from build123d import *

# Parameters (mm, degrees)
F0_W     = 5
F0_H     = 50
F0_W_2   = 138.5
F0_H_2   = 20
F0_W_3   = 50
F0_H_3   = 5
F0_H_4   = 4
F0_W_4   = 20
F0_W_5   = 4
F0_H_5   = 175
F0_W_6   = 40
F0_H_6   = 40
F0_R     = 20
F1_DEPTH = 1
F0_W_7   = 128.5
F0_H_7   = 147
F2_DEPTH = 1
F3_W     = 6
F3_H     = 6
F4_DEPTH = 25


with BuildPart() as f1:
    # F0 (on Top) → F1 (new body)
    with BuildSketch(Plane.XY):
        with Locations((-231, -87.5)):
            Rectangle(F0_W, F0_H)
        with Locations((-69.25, -122.5)):
            Rectangle(F0_W_2, F0_H_2)
        with Locations((-183.5, -40)):
            Rectangle(F0_W_3, F0_H_3)
        with Locations((-69.25, 114.5)):
            Rectangle(F0_W_2, F0_H_4)
        with Locations((-218.5, -87.5)):
            Rectangle(F0_W_4, F0_H)
        with Locations((-183.5, -52.5)):
            Rectangle(F0_W_3, F0_H_2)
        with Locations((-140.5, 25)):
            Rectangle(F0_W_5, F0_H_5)
        Polygon((-138.5, -112.5), (-138.5, -62.5), (-142.5, -62.5), (-158.5, -62.5), (-158.5, -112.5), align=None)
        with Locations((-183.5, -87.5)):
            Rectangle(F0_W_3, F0_H)
        with Locations((-183.5, -87.5)):
            Rectangle(F0_W_6, F0_H_6, mode=Mode.SUBTRACT)
        Polygon((0, 102.5), (0, 112.5), (-138.5, 112.5), (-138.5, -62.5), (-138.5, -112.5), (0, -112.5), (0, -44.5), (-128.5, -44.5), (-128.5, 102.5), align=None)
        with Locations((-113.5, -87.5)):
            Circle(F0_R, mode=Mode.SUBTRACT)
    extrude(amount=F1_DEPTH)

    # F0 (on Top) → F2 (join)
    with BuildSketch(Plane.XY):
        Polygon((0, 102.5), (0, 112.5), (-138.5, 112.5), (-138.5, -62.5), (-138.5, -112.5), (0, -112.5), (0, -44.5), (-128.5, -44.5), (-128.5, 102.5), align=None)
        with Locations((-113.5, -87.5)):
            Circle(F0_R, mode=Mode.SUBTRACT)
        with Locations((-69.25, 114.5)):
            Rectangle(F0_W_2, F0_H_4)
        with Locations((-140.5, 25)):
            Rectangle(F0_W_5, F0_H_5)
        with Locations((-64.25, 29)):
            Rectangle(F0_W_7, F0_H_7)
        Polygon((-138.5, -112.5), (-138.5, -62.5), (-142.5, -62.5), (-158.5, -62.5), (-158.5, -112.5), align=None)
        with Locations((-69.25, -122.5)):
            Rectangle(F0_W_2, F0_H_2)
        with Locations((-183.5, -87.5)):
            Rectangle(F0_W_3, F0_H)
        with Locations((-183.5, -87.5)):
            Rectangle(F0_W_6, F0_H_6, mode=Mode.SUBTRACT)
        with Locations((-183.5, -52.5)):
            Rectangle(F0_W_3, F0_H_2)
        with Locations((-218.5, -87.5)):
            Rectangle(F0_W_4, F0_H)
        with Locations((-183.5, -40)):
            Rectangle(F0_W_3, F0_H_3)
        with Locations((-231, -87.5)):
            Rectangle(F0_W, F0_H)
    extrude(amount=F2_DEPTH)

    # F3 (on face) → F4 (cut)
    with BuildSketch(Plane.XY.offset(1)):
        with Locations((-138.5, -112.5)):
            Rectangle(F3_W, F3_H)
        with Locations((-158.5, -62.5)):
            Rectangle(F3_W, F3_H)
        with Locations((-208.5, -62.5)):
            Rectangle(F3_W, F3_H)
        with Locations((-138.5, 112.5)):
            Rectangle(F3_W, F3_H)
    extrude(amount=-F4_DEPTH, mode=Mode.SUBTRACT)


solid = f1.part
Verification items for the finished model (mm, model axes). Coordinates: 2 decimals unless noted, no trailing zeros. Order: outer loops, then holes, each group sorted by start corner. A loop starts at its lowest first (then second) coordinate and runs counter-clockwise, first axis right, second up.
Item 1: Section check B-B, the plane x = -113.5. Enter the section's corners in (y, z).
Filled in:
outline: (-132.5, 0) - (-107.5, 0) - (-107.5, 1) - (-132.5, 1) - close; (-67.5, 0) - (116.5, 0) - (116.5, 1) - (-67.5, 1) - close
Item 2: Depth check by flat-ended pin: pin 1 (0.5 mm diameter, centred on x = -207.5, z = 0.5, fed in from +Y); pin 2 (0.5 mm diameter, centred on y = -113, z = 0.5, fed in from -X); pin 3 (0.5 mm diameter, centred on x = -207, z = 0.5, fed in from -Y); pin 4 (8 mm diameter, centred on x = -82, y = -71, fed in from -Z). Enter the tip coordinate at first touch or a pass-through.
Filled in:
pin 1: stops at y = -37.5
pin 2: stops at x = -135.5
pin 3: stops at y = -112.5
pin 4: stops at z = 0
Item 3: Material ranges on L1, parallel to Y at x = -138, z = 0.45; L2, parallel to Y at x = -113.5, z = 0.4; L3, parallel to X at y = 24, z = 0.5, recorded low to high.
Filled in:
L1: y = -132.5 to -115.5, -109.5 to 109.5, 115.5 to 116.5
L2: y = -132.5 to -107.5, -67.5 to 116.5
L3: x = -142.5 to 0
Item 4: Section check A-A, the plane y = -47.5. Enter the section's corners in (x, z).
Filled in:
outline: (-208.5, 0) - (-158.5, 0) - (-158.5, 1) - (-208.5, 1) - close; (-142.5, 0) - (0, 0) - (0, 1) - (-142.5, 1) - close
Item 5: Release check for a two-part mould opening along X. For faces 1 (the face through (-129.37, -99.67, 0.49)), 2 (the face through (-66, -6, 1)) record: +X half, -X half, draft (parallel to the pull), parting line (faces both ways), or undercut.
Filled in:
face 1: undercut
face 2: draft
Item 6: Section check C-C, the plane y = -87.5. Enter the section's corners in (x, z), then the cut area to 4 significant figures.
Filled in:
outline: (-233.5, 0) - (-203.5, 0) - (-203.5, 1) - (-233.5, 1) - close; (-163.5, 0) - (-133.5, 0) - (-133.5, 1) - (-163.5, 1) - close; (-93.5, 0) - (0, 0) - (0, 1) - (-93.5, 1) - close
area: 153.5 mm2
Item 7: Section check D-D, the plane z = 0.3. Give the number of separate pieces and of enclosed holes in the cut face, then the cut area to 3 significant figures.
Filled in:
separate pieces: 1
enclosed holes: 2
area: 38,200 mm2
